Geometry: final body of the model. Coordinates: model frame, mm. Give positions to 0.01 mm unless a question says otherwise; leave off trailing zeros. Order: outer loops, then holes, each group sorted by start corner. A loop starts at its lowest first (then second) coordinate and runs counter-clockwise, first axis right, second up. Notation, with made-up numbers: (-26, -28) -> (12, -28) arc R19 cw to (12, 1) -> close; hole circle Ø1 at (-27.75, -10). An arc over 180 degrees is marked (long way). One line per question, with ' | ' between items.
from build123d import *

# Parameters (mm, degrees)
F1_DEPTH = 317.5
F2_R     = 2.54
F3_R     = 2.54


with BuildPart() as f1:
    # F0 (on Top) → F1 (new body)
    with BuildSketch(Plane.XY):
        with BuildLine():
            Line((-8.061039, 7.452499), (-8.061039, 0))
            Line((-8.061039, 0), (-8.061039, -2.707501))
            ThreePointArc((-8.061039, -2.707501), (-0.441039, -10.327501), (7.178961, -2.707501))
            Line((7.178961, -2.707501), (7.178961, 0))
            Line((7.178961, 0), (7.178961, 7.452499))
            ThreePointArc((7.178961, 7.452499), (-0.441039, 15.072499), (-8.061039, 7.452499))
        make_face()
    extrude(amount=F1_DEPTH)

    # F2
    f2_edges = [f1.edges().sort_by_distance(p)[0] for p in [
        (-0.441039, 15.072499, 317.5),
        (7.178961, 2.372499, 317.5),
        (-0.441039, -10.327501, 317.5),
        (-8.061039, 2.372499, 317.5),
    ]]
    fillet(f2_edges, radius=F2_R)

    # F3
    f3_edges = [f1.edges().sort_by_distance(p)[0] for p in [
        (-0.441039, 15.072499, 0),
        (-0.441039, -10.327501, 0),
        (7.178961, 2.372499, 0),
        (-8.061039, 2.372499, 0),
    ]]
    fillet(f3_edges, radius=F3_R)


solid = f1.part
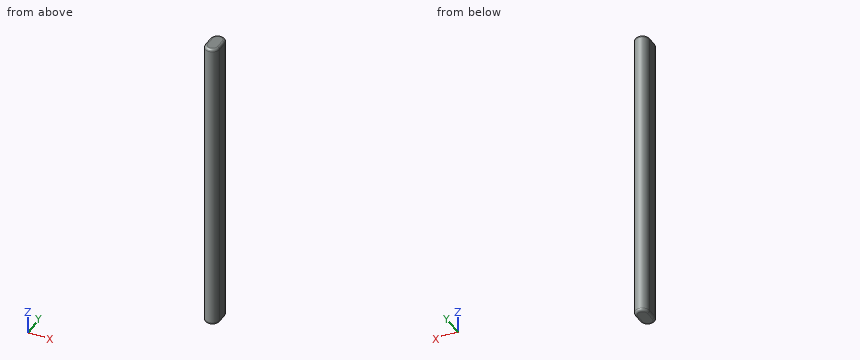
1) Material intervals for probe 1 along Z at (x, y) = (4, -5.5); probe 2 along Y at (x, z) = (0.5, 241.5); probe 3 along Y at (x, z) = (-0.75, 16), sorted ascending. Write a range as from..to.
Check result:
probe 1: z = 0.01..317.49 | probe 2: y = -10.27..15.01 | probe 3: y = -10.32..15.07
2) Contact query for a flat-ended pin moving along its axis: pin 1 Ø3 at (x, z) = (-5, 52.5) entering from -Y. Output: stop coordinate, or through.
Check result:
pin 1: stops at y = -9.69
3) Section A-A on z = 213. Return loops of the section in (x, y).
Check result:
outline: (-8.06, -2.71) arc R7.62 ccw to (7.18, -2.71) -> (7.18, 7.45) arc R7.62 ccw to (-8.06, 7.45) -> close
